The figure shows three views and two pictorial views of one solid part (mm, origin at its lowest corner). Answer the questions. Coordinates: 2 decimals unless noted, no trailing zeros. Order: outer loops, then holes, each group sorted by start corner. A loop starts at its lowest first (then second) coordinate and runs counter-clockwise, first axis right, second up. Notation, with made-up numbers: (-4.5, -29.75) -> (40.5, -29.75) arc R20 ccw to (40.5, -12.75) -> close; hole circle Ø8 at (56, 8.5). An arc over 180 degrees is marked (long way). Write item = value, one per line. Start each with the question number.
Q1. Straight lines are drawn through the part: L1, parallel to X at y = 163, z = 0.15; L2, parallel to X at y = 157, z = 0.7. For each, find the intervals that lie inside material, in ascending order. Write a range as from..to.
Q2. The part is cut by section B-B, the plane x = 27. Determine the outline of the cut face in (y, z).
Q3. The part is cut by section A-A, the plane z = 1.65. Count the separate pieces of the cut face and the enclosed holes in it, plus the area to 3 significant figures.
Q4. Flat-ended cylindrical pins translate along their axes: pin 1 (1 mm diameter, centred on y = 79.5, z = 2, fed in from +X); pin 2 (2 mm diameter, centred on x = 128, y = 4, fed in from +Z). Find the tip coordinate at first contact, or state that the pin passes through.
Q5. The part is cut by section C-C, the plane y = 153. Determine the outline of the cut face in (x, z), plus the area to 3 significant figures.
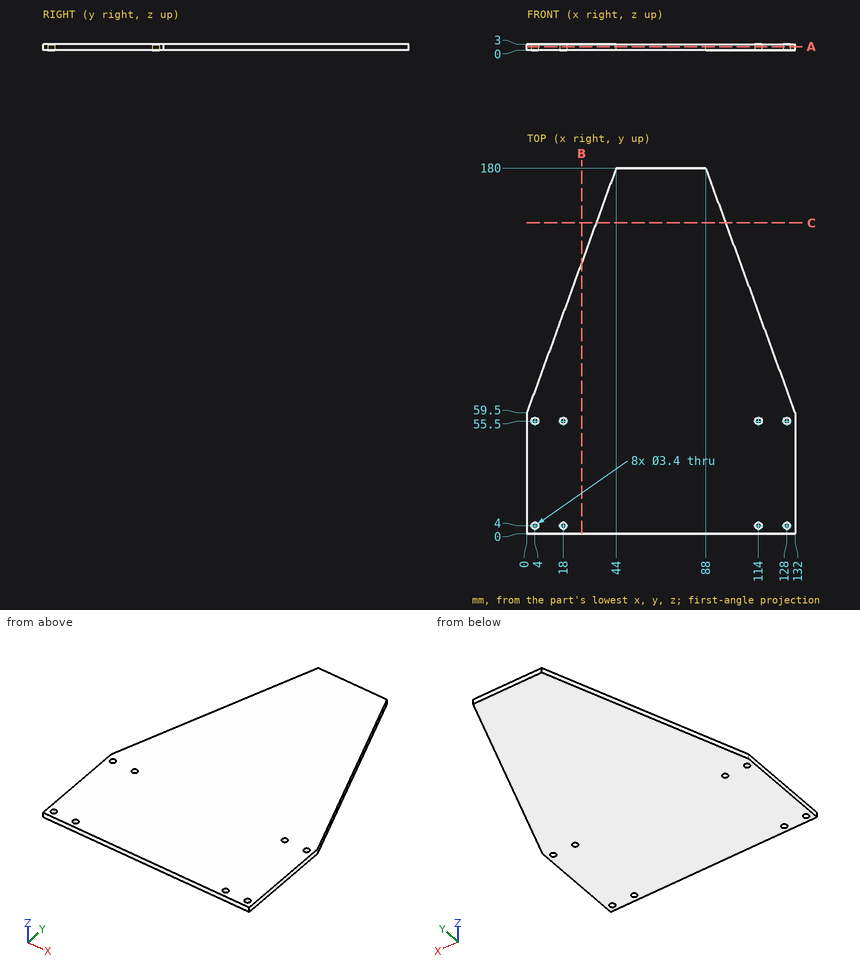
Model answer:
q1.L1 = 37.79..94.21
q1.L2 = 35.6..96.4
q2.outline = (0, 0) -> (133.44, 0) -> (133.44, 3) -> (0, 3) -> close
q3.separate_pieces = 1
q3.enclosed_holes = 8
q3.area = 18,400 mm2
q4.pin_1 = 124.88
q4.pin_2 = through
q5.outline = (34.14, 0) -> (97.86, 0) -> (97.86, 3) -> (34.14, 3) -> close
q5.area = 191 mm2
